from build123d import *

# Parameters (mm, degrees)
SKETCH2_R           = 3.175
BOSS_EXTRUDE1_DEPTH = 7.62
BOSS_EXTRUDE2_DEPTH = 5.58
FILLET1_R           = 5.08
FILLET3_R           = 1.27
SKETCH4_RX          = 64.751719118
SKETCH4_RY          = 35.535243055
CUT_EXTRUDE1_DEPTH  = 8.89


with BuildPart() as part:
    # Sketch2 → Boss-Extrude1 (new body)
    with BuildSketch(Plane(origin=(0, 0, 0), x_dir=(0, 0, -1), z_dir=(1, 0, 0))):
        with BuildLine():
            ThreePointArc((3.174202727, -63.420615237), (63.5, 0), (3.174202727, 63.420615237))
            ThreePointArc((3.174202727, 63.420615237), (0.000185525, 60.324999039), (-3.173812636, 63.42063476))
            ThreePointArc((-3.173812636, 63.42063476), (-63.5, 0), (-3.173812636, -63.42063476))
            ThreePointArc((-3.173812636, -63.42063476), (0.000185525, -60.324999039), (3.174202727, -63.420615237))
        make_face()
        with Locations(Location((0, 0, 0), (0, 0, 180))):
            Circle(SKETCH2_R, mode=Mode.SUBTRACT)
    extrude(amount=BOSS_EXTRUDE1_DEPTH)

    # Sketch3 → Boss-Extrude2 (add)
    with BuildSketch(Plane(origin=(7.62, 0, 0), x_dir=(0, 0, -1), z_dir=(1, 0, 0))):
        Polygon((19.05, -10.998522628), (0, 21.997045256), (-19.05, -10.998522628), align=None)
        Polygon((-5.675, 3.276462778), (-5.675, -3.276462778), (0, -6.552925555), (5.675, -3.276462778), (5.675, 3.276462778), (0, 6.552925555), align=None, mode=Mode.SUBTRACT)
    extrude(amount=BOSS_EXTRUDE2_DEPTH)

    # Fillet1
    fillet1_edges = [part.edges().sort_by_distance(p)[0] for p in [
        (10.41, -10.998522628, 19.05),
        (10.41, -10.998522628, -19.05),
        (10.41, 21.997045256, 0),
    ]]
    fillet(fillet1_edges, radius=FILLET1_R)

    # Fillet3
    fillet3_edges = [part.edges().sort_by_distance(p)[0] for p in [
        (7.62, 0, -63.5),
        (7.62, 0, 63.5),
    ]]
    fillet(fillet3_edges, radius=FILLET3_R)

    # Sketch4 → Cut-Extrude1 (cut)
    with BuildSketch(Plane.ZY):
        with Locations(Location((-63.5, 0), (0, 0, -90))):
            Ellipse(SKETCH4_RX, SKETCH4_RY)
    cut_extrude1 = extrude(amount=-CUT_EXTRUDE1_DEPTH, mode=Mode.SUBTRACT)

    # Mirror1: Cut-Extrude1 across plane
    add(cut_extrude1.mirror(Plane.XY), mode=Mode.SUBTRACT)


solid = part.part
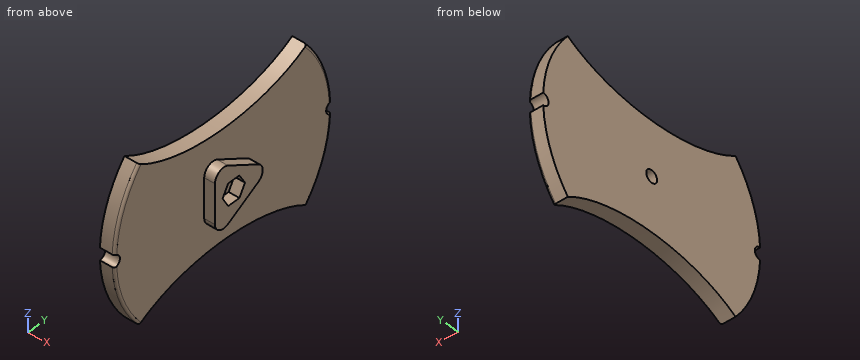
The listing builds one solid part. Answer for the finished solid, in the listing's coordinates (mm). Round coordinates to 2 decimals unless told otherwise and drop trailing zeros. Order: outer loops, then holes, each group sorted by start corner. A loop starts at its lowest first (then second) coordinate and runs counter-clockwise, first axis right, second up. Notation, with made-up numbers: M 46,53.5 L 71,53.5 A24 ccw 71,82.5 Z; hole C -34.75,36.5 d11. An arc over 180 degrees is marked long. Answer in a Markdown table with one row per item. Add a question column.
1) The part is cut by section A-A on x = 10. Determine the outline of the cut face in (y, z) (3 decimals).
2) Consider line 1 along Y through (x, z) = (2.75, 0) (3 decimals); line 2 along X through (y, z) = (0.5, 5); line 3 along Y through (x, z) = (2.5, -18). Determine where each line is inside the solid, lowest interval first. Write a range as from..to.
3) Flat-ended cylindrical pins translate along their axes: pin 1 Ø5 at (y, z) = (-29.5, -11) entering from +X; pin 2 Ø5 at (x, z) = (4, 21.5) entering from -Y; pin 3 Ø1.7 at (x, y) = (11, -0.5) entering from -Z. Find the tip coordinate at first contact, or state that the pin passes through.
Findings below:
| question | item | result |
|---|---|---|
| 1 | outline | M -10.999,-10.251 A5.08 ccw -3.379,-14.651 L 14.377,-4.399 A5.08 ccw 14.377,4.399 L -3.379,14.651 A5.08 ccw -10.999,10.251 Z; hole M -6.553,0 L -3.276,-5.675 L 3.276,-5.675 L 6.553,0 L 3.276,5.675 L -3.276,5.675 Z |
| 2 | line 1 | y = -60.325..-3.175, 3.175..60.325 |
| 2 | line 2 | x = 0..7.62 |
| 2 | line 3 | y = -60.9..60.9 |
| 3 | pin 1 | stops at x = 7.62 |
| 3 | pin 2 | stops at y = -60.59 |
| 3 | pin 3 | stops at z = -13.48 |
